CAD build for the part. Positions are in the model's coordinates, mm. A direction names the side the tool comes from. Give positions to 0.01 mm unless a question says otherwise; leave off trailing zeros. Loops run counter-clockwise (first coordinate to the right, second up) from the corner with the lowest first, then second, coordinate; pieces in that order, holes last.
Item 1: Saw through at D-D on y = -15.5. Give the cut face in (x, z).
Item 2: Saw through at A-A on y = 24. Give the cut face in (x, z), plus the area to 3 significant figures.
Item 3: Mould opens along Y. For faces 1 (the flat face through (-50.8, 0, 13)), 2 (the flat face through (31, -3, 25.4)), 3 (the cylindrical face through (48.01, 7.44, 12.88)) say: released by +Y, released by -Y, zero draft, split by the parting line, or undercut.
Item 4: Saw through at C-C on x = 1. Give the cut face in (y, z), plus the area to 3 significant figures.
Item 5: Which spindle directions (+Z, -Z, +X, -X, +Y, -Y) get a long thin tool onto all of the face, cutting with end or side? Do faces 4 (the cylindrical face through (56.65, -25.71, 12.52)), 5 (the flat face through (74.818, 22.231, 12.878)), 6 (the flat face through (-28, -8.89, 13)), 7 (the flat face through (-55, 8.89, 13)). Say none if no direction does.
Item 6: Drop flat-ended pins along their axis: P1, Ø3, axis at x = -54, z = 9, coming from the +Y side; P2, Ø9, axis at x = 59, z = 8.5, coming from the +Y side; P3, Ø0.5, axis at y = 3, z = 14, coming from the +X side; P4, Ø5, axis at x = 65, y = 13.5, coming from the -Z side. Give the stop position or say it passes through.
Item 7: Probe probe 1 along Y at (x, z) = (-41, 7); probe 2 along X at (y, z) = (17, 3.75); probe 3 along Y at (x, z) = (74.5, 7.5). List the from-to ranges inside material, lowest first.
from build123d import *

# Parameters (mm, degrees)
F1_DEPTH = 25.4
F3_DEPTH = 25.4
F4_R     = 25.4
F5_R     = 5.07999
F6_R     = 1.524
F7_DEPTH = 25.4


# Not quite as in the source:
# - a fillet or chamfer is up to 0.001 mm smaller than in the source, because OpenCascade refuses the exact size


with BuildPart() as f1:
    # F0 (on Top) → F1 (new body)
    with BuildSketch(Plane.XY):
        Polygon((-46.482, 8.89), (-62.992, 8.89), (-62.992, -8.89), (62.992, -8.89), (62.992, 8.89), (46.482, 8.89), (46.482, 3.81), (56.642, 3.81), (56.642, 1.9812), (50.8, 1.9812), (50.8, -2.7178), (-50.8, -2.7178), (-50.8, 1.9812), (-56.642, 1.9812), (-56.642, 3.81), (-46.482, 3.81), align=None)
    extrude(amount=F1_DEPTH)

    # F2 (on face) → F3 (join)
    with BuildSketch(Plane.XY.offset(25.4)):
        Polygon((75.6565171085, 36.049144584), (62.992, 8.89), (62.992, -8.89), (3.4387046284, -8.89), (60.5084189693, -35.5020448459), (90.6196586724, 29.0717170827), (86.0156151143, 31.2186178523), (75.2811112661, 8.1984000616), (69.5260568184, 10.8820260237), (80.2605606666, 33.9022438144), align=None)
    extrude(amount=-F3_DEPTH)

    # F4
    f4_edges = [f1.edges().sort_by_distance(p)[0] for p in [
        (60.508419, -35.502045, 12.7),
    ]]
    fillet(f4_edges, radius=F4_R)

    # F5 (radius 5.08 in the source; OpenCascade refuses exactly that, so slightly less here)
    f5_edges = [f1.edges().sort_by_distance(p)[0] for p in [
        (-62.992, -8.89, 12.7),
        (-62.992, 8.89, 12.7),
        (75.656517, 36.049145, 12.7),
        (46.482, 8.89, 12.7),
        (-46.482, 8.89, 12.7),
    ]]
    fillet(f5_edges, radius=F5_R)

    # F6 (on face) → F7 (cut)
    with BuildSketch(Plane(origin=(48.336171005, -22.5395267055, 0), x_dir=(-0.4226182617, -0.906307787, 0), z_dir=(-0.906307787, 0.4226182617, 0))):
        with Locations((-47.1220459863, 12.7)):
            Circle(F6_R)
    extrude(amount=-F7_DEPTH, mode=Mode.SUBTRACT)


solid = f1.part
Results below:
1. outline: (17.61, 0) - (69.58, 0) - (69.58, 25.4) - (17.61, 25.4) - close
2. outline: (70.04, 0) - (75.64, 0) - (75.64, 25.4) - (70.04, 25.4) - close; (82.65, 0) - (88.25, 0) - (88.25, 25.4) - (82.65, 25.4) - close
2. area: 285 mm2
3. face 1: undercut
3. face 2: zero draft
3. face 3: released by +Y
4. outline: (-8.89, 0) - (-2.72, 0) - (-2.72, 25.4) - (-8.89, 25.4) - close
4. area: 157 mm2
5. face 4: +Z, -Z, -Y
5. face 5: +Z, -Z
5. face 6: +Z, -Z, -X, -Y
5. face 7: +Z, -Z, -X, +Y
6. P1: stops at y = 8.89
6. P2: stops at y = 9.98
6. P3: stops at x = 78.58
6. P4: stops at z = 0
7. probe 1: y = -8.89 to -2.72
7. probe 2: x = 66.77 to 72.38, 79.39 to 84.99
7. probe 3: y = -5.5 to 8.56, 21.55 to 32.87
